from build123d import *

# Parameters (mm, degrees)
F0_W     = 138.5714327227
F0_H     = 50
F1_DEPTH = 50
F2_R     = 5
F3_DEPTH = 50.001
F5_DEPTH = 50.001
F7_DEPTH = 50.001
F9_DEPTH = 25


with BuildPart() as f1:
    # F0 (on Front) → F1 (new body)
    with BuildSketch(Plane.XZ):
        with Locations((1.709715571, -25)):
            Rectangle(F0_W, F0_H)
    extrude(amount=F1_DEPTH)

    # F2 (on face) → F3 (cut, through all)
    with BuildSketch(Plane.XZ):
        with Locations((-61.9109951626, -5.7210989713)):
            Circle(F2_R)
        with Locations((-61.9109951626, -18.7210989713)):
            Circle(F2_R)
        with Locations((-61.9109951626, -31.7210989713)):
            Circle(F2_R)
        with Locations((-61.9109951626, -44.7210989713)):
            Circle(F2_R)
        with Locations((-50.4109951626, -5.7210989713)):
            Circle(F2_R)
        with Locations((-50.4109951626, -18.7210989713)):
            Circle(F2_R)
        with Locations((-50.4109951626, -31.7210989713)):
            Circle(F2_R)
        with Locations((-50.4109951626, -44.7210989713)):
            Circle(F2_R)
        with Locations((-38.9109951626, -5.7210989713)):
            Circle(F2_R)
        with Locations((-38.9109951626, -18.7210989713)):
            Circle(F2_R)
        with Locations((-38.9109951626, -31.7210989713)):
            Circle(F2_R)
        with Locations((-38.9109951626, -44.7210989713)):
            Circle(F2_R)
        with Locations((-27.4109951626, -5.7210989713)):
            Circle(F2_R)
        with Locations((-27.4109951626, -18.7210989713)):
            Circle(F2_R)
        with Locations((-27.4109951626, -31.7210989713)):
            Circle(F2_R)
        with Locations((-27.4109951626, -44.7210989713)):
            Circle(F2_R)
        with Locations((-15.9109951626, -5.7210989713)):
            Circle(F2_R)
        with Locations((-15.9109951626, -18.7210989713)):
            Circle(F2_R)
        with Locations((-15.9109951626, -31.7210989713)):
            Circle(F2_R)
        with Locations((-15.9109951626, -44.7210989713)):
            Circle(F2_R)
        with Locations((-4.4109951626, -5.7210989713)):
            Circle(F2_R)
        with Locations((-4.4109951626, -18.7210989713)):
            Circle(F2_R)
        with Locations((-4.4109951626, -31.7210989713)):
            Circle(F2_R)
        with Locations((-4.4109951626, -44.7210989713)):
            Circle(F2_R)
        with Locations((7.0890048374, -5.7210989713)):
            Circle(F2_R)
        with Locations((7.0890048374, -18.7210989713)):
            Circle(F2_R)
        with Locations((7.0890048374, -31.7210989713)):
            Circle(F2_R)
        with Locations((7.0890048374, -44.7210989713)):
            Circle(F2_R)
        with Locations((18.5890048374, -5.7210989713)):
            Circle(F2_R)
        with Locations((18.5890048374, -18.7210989713)):
            Circle(F2_R)
        with Locations((18.5890048374, -31.7210989713)):
            Circle(F2_R)
        with Locations((18.5890048374, -44.7210989713)):
            Circle(F2_R)
        with Locations((30.0890048374, -5.7210989713)):
            Circle(F2_R)
        with Locations((30.0890048374, -18.7210989713)):
            Circle(F2_R)
        with Locations((30.0890048374, -31.7210989713)):
            Circle(F2_R)
        with Locations((30.0890048374, -44.7210989713)):
            Circle(F2_R)
        with Locations((41.5890048374, -5.7210989713)):
            Circle(F2_R)
        with Locations((41.5890048374, -18.7210989713)):
            Circle(F2_R)
        with Locations((41.5890048374, -31.7210989713)):
            Circle(F2_R)
        with Locations((41.5890048374, -44.7210989713)):
            Circle(F2_R)
        with Locations((53.0890048374, -5.7210989713)):
            Circle(F2_R)
        with Locations((53.0890048374, -18.7210989713)):
            Circle(F2_R)
        with Locations((53.0890048374, -31.7210989713)):
            Circle(F2_R)
        with Locations((53.0890048374, -44.7210989713)):
            Circle(F2_R)
        with Locations((64.5890048374, -5.7210989713)):
            Circle(F2_R)
        with Locations((64.5890048374, -18.7210989713)):
            Circle(F2_R)
        with Locations((64.5890048374, -31.7210989713)):
            Circle(F2_R)
        with Locations((64.5890048374, -44.7210989713)):
            Circle(F2_R)
    extrude(amount=F3_DEPTH, mode=Mode.SUBTRACT)

    # F4 (on face) → F5 (cut, through all)
    with BuildSketch(Plane.XY):
        Polygon((37.2054319323, 0), (-33.7860007904, 0), (0, -20), align=None)
    extrude(amount=-F5_DEPTH, mode=Mode.SUBTRACT)

    # F6 (on face) → F7 (cut, through all)
    with BuildSketch(Plane.XY):
        Polygon((0, -50), (-67.5760007904, -25), (-67.5760007904, -50), align=None)
        Polygon((70.9954319323, -25), (0, -50), (70.9954319323, -50), align=None)
    extrude(amount=-F7_DEPTH, mode=Mode.SUBTRACT)

    # F8 (on face) → F9 (cut)
    with BuildSketch(Plane.XY):
        Polygon((-67.5760007904, 0), (-67.5760007904, -25), (-33.7860007904, 0), align=None)
        Polygon((37.2054319323, 0), (70.9954319323, -25), (70.9954319323, 0), (39.7841334343, 0), align=None)
    extrude(amount=-F9_DEPTH, mode=Mode.SUBTRACT)


solid = f1.part
The listing builds one solid part. Answer for the finished solid, in the listing's coordinates (mm). A direction names the side the tool comes from. Give positions to 0.01 mm unless a question says otherwise; leave off trailing zeros. Order: outer loops, then holes, each group sorted by start corner. A loop starts at its lowest first (then second) coordinate and runs counter-clockwise, first axis right, second up. Notation, with made-up numbers: (-38, 7.25) - (20, 7.25) arc R26 cw to (20, 36.25) - close; hole circle Ø6 at (48, 24). An arc over 180 degrees is marked (long way). Use one line per item in the form item = value.
1) Each of these flat-tipped pins is pushed along its axis until it touches: pin 1 (13 mm diameter, centred on x = -27.41, z = -18.72, fed in from -Y); pin 2 (6 mm diameter, centred on x = 25.5, z = -20.5, fed in from +Y); pin 3 (10 mm diameter, centred on x = 12, z = -15.5, fed in from -Y). Where does it stop, or does it pass through?
Verdict:
pin_1 = -42.26
pin_2 = -5.31
pin_3 = -47.42
2) For faces 4 (the flat face through (61, -7, -25)), 5 (the cylindrical face through (-22.64, -20.91, -4.22)), determine the directions among +Z, -Z, +X, -X, +Y, -Y from which every point of the face is accessible in a straight line to the end or side of a thin tool.
Verdict:
face_4 = +Z, +X, +Y
face_5 = +Y, -Y
3) Find section C-C on y = -39.5. Give the number of separate pieces and of enclosed holes in the cut face, and give its area (3 significant figures).
Verdict:
separate_pieces = 1
enclosed_holes = 16
area = 1,310 mm^2
4) Find section A-A on x = -18.5. Determine the outline of the cut face in (y, z).
Verdict:
outline = (-43.16, -50) - (-9.05, -50) - (-9.05, -49) - (-43.16, -49) - close; (-43.16, -40.44) - (-9.05, -40.44) - (-9.05, -36) - (-43.16, -36) - close; (-43.16, -27.44) - (-9.05, -27.44) - (-9.05, -23) - (-43.16, -23) - close; (-43.16, -14.44) - (-9.05, -14.44) - (-9.05, -10) - (-43.16, -10) - close; (-43.16, -1.44) - (-9.05, -1.44) - (-9.05, 0) - (-43.16, 0) - close
5) Find section B-B on x = -52.5. Determine the outline of the cut face in (y, z).
Verdict:
outline = (-30.58, -50) - (0, -50) - (0, -49.26) - (-30.58, -49.26) - close; (-30.58, -40.18) - (0, -40.18) - (0, -36.26) - (-30.58, -36.26) - close; (-30.58, -27.18) - (0, -27.18) - (0, -25) - (-13.85, -25) - (-13.85, -23.26) - (-30.58, -23.26) - close; (-30.58, -14.18) - (-13.85, -14.18) - (-13.85, -10.26) - (-30.58, -10.26) - close; (-30.58, -1.18) - (-13.85, -1.18) - (-13.85, 0) - (-30.58, 0) - close
6) Consider probe 1 along Z at (x, y) = (-38.5, -20); probe 2 along Z at (x, y) = (37, -6.5); probe 3 along Y at (x, z) = (50, -27). Determine where each line is inside the solid, lowest interval first. Write a range as [from, to].
Verdict:
probe_1 = [-50, -49.7], [-39.74, -36.7], [-26.74, -23.7], [-13.74, -10.7], [-0.74, 0]
probe_2 = [-50, -46.71], [-42.74, -33.71], [-29.74, -20.71], [-16.74, -7.71], [-3.74, 0]
probe_3 = [-32.39, 0]
7) The mould has two halves that part along X. Classify faces 1 (the cylindrical face through (-45.792, -16.368, -33.636)), 2 (the flat face through (1, -25, 0)), 3 (the flat face through (-50.918, -12.675, -12.325)): released by +X, released by -X, zero draft, split by the parting line, or undercut.
Verdict:
face_1 = undercut
face_2 = zero draft
face_3 = released by -X
8) Find section D-D on x = 20. Determine the outline of the cut face in (y, z), and give its area (3 significant figures).
Verdict:
outline = (-42.96, -50) - (-9.25, -50) - (-9.25, -49.52) - (-42.96, -49.52) - close; (-42.96, -39.92) - (-9.25, -39.92) - (-9.25, -36.52) - (-42.96, -36.52) - close; (-42.96, -26.92) - (-9.25, -26.92) - (-9.25, -23.52) - (-42.96, -23.52) - close; (-42.96, -13.92) - (-9.25, -13.92) - (-9.25, -10.52) - (-42.96, -10.52) - close; (-42.96, -0.92) - (-9.25, -0.92) - (-9.25, 0) - (-42.96, 0) - close
area = 392 mm^2
